Autodesk Inventor part; units mm, degrees
ref_plane "YZ Plane" through (0, 0, 0) normal (1, 0, 0) x (0, 1, 0)
ref_plane "XZ Plane" through (0, 0, 0) normal (0, 1, 0) x (-1, 0, 0)
ref_plane "XY Plane" through (0, 0, 0) normal (0, 0, 1) x (1, 0, 0)
sketch "Sketch1" plane through (0, 0, 0) normal (1, 0, 0) x (0, 1, 0)
  line L0 (0, 0) -> (0, -6)
  arc A0 (-0.5, -6.866) -> (0, -6) centre (-1, -6) ccw
  arc A1 (-0.5, -6.866) -> (-1.1, -7.9053) centre (0.1, -7.9053) ccw
  line L1 (-1.1, -7.9053) -> (-1.1, -13.9053)
  line L2 (-1.1, -13.9053) -> (-0.9, -13.9053)
  line L3 (-0.9, -13.9053) -> (-0.9, -7.9053)
  arc A2 (-0.4, -7.0392) -> (-0.9, -7.9053) centre (0.1, -7.9053) ccw
  arc A3 (-0.4, -7.0392) -> (0.2, -6) centre (-1, -6) ccw
  line L4 (0.2, -6) -> (0.2, 0)
  line L5 (0.2, 0) -> (0, 0)
  dimension "d0" = 0.2
  dimension "d1" = 6
  dimension "d2" = 6
  dimension "d3" = 1.1
  dimension "d4" = 1
extrude "Extrusion1" add sketch "Sketch1" along normal mid plane 2
properties part number "SolarPanel_CellJumper" material "Nickel-Copper Alloy 400"
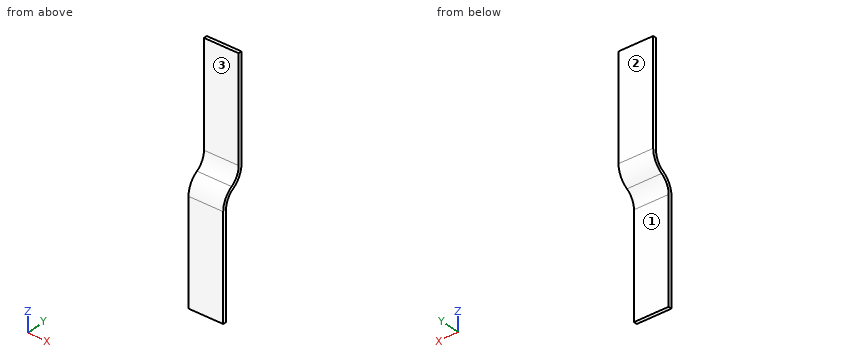
Work out the finished part from the listing and answer in its coordinate system (mm). Face numbers are marked on the shaded views. A direction names the side the tool comes from. Round coordinates to 2 decimals unless told otherwise and drop trailing zeros. Order: outer loops, then holes, each group sorted by start corner. A loop starts at its lowest first (then second) coordinate and runs counter-clockwise, first axis right, second up. Notation, with made-up numbers: M 41.5,34 L 69.5,34 A26 cw 69.5,70 Z; hole C -33,18 d10. An arc over 180 degrees is marked long. Put each result on its own line as item: value. Start each with the question number.
Q1. Straight lines are drawn through the part: L1, parallel to Y at x = 0.55, z = -1.5; L2, parallel to Y at x = 0.55, z = -11.5; L3, parallel to Z at x = 0.45, y = -0.95. For each, find the intervals that lie inside material, in ascending order. Write a range as [from, to].
Q2. Section C-C, the plane y = -0.2 is taken. Write down the section's boundary in (x, z), and give its area (3 significant figures).
Q3. Section A-A, the plane x = 0.3 is taken. Write down the section's boundary in (y, z), and give its area (3 significant figures).
Q4. A tool of negligible diameter and unlimited length cuts with its end or side. For the marked faces 1, 2 and 3, from which of +Z, -Z, +X, -X, +Y, -Y can it reach the whole face along a straight path? Write none if from no direction.
Q5. Section B-B, the plane z = -10.5 is taken. Write down the section's boundary in (x, y).
Findings below:
1. L1: y = [0, 0.2]
1. L2: y = [-1.1, -0.9]
1. L3: z = [-13.91, -7.32]
2. outline: M -1,-6.89 L 1,-6.89 L 1,-6.6 L -1,-6.6 Z
2. area: 0.589 mm^2
3. outline: M -1.1,-13.91 L -0.9,-13.91 L -0.9,-7.91 A1 cw -0.4,-7.04 A1.2 ccw 0.2,-6 L 0.2,0 L 0,0 L 0,-6 A1 cw -0.5,-6.87 A1.2 ccw -1.1,-7.91 Z
3. area: 2.86 mm^2
4. face 1: -Z, +X, -X, +Y
4. face 2: +Z, -Z, +X, -X, +Y
4. face 3: +Z, +X, -X, -Y
5. outline: M -1,-1.1 L 1,-1.1 L 1,-0.9 L -1,-0.9 Z
